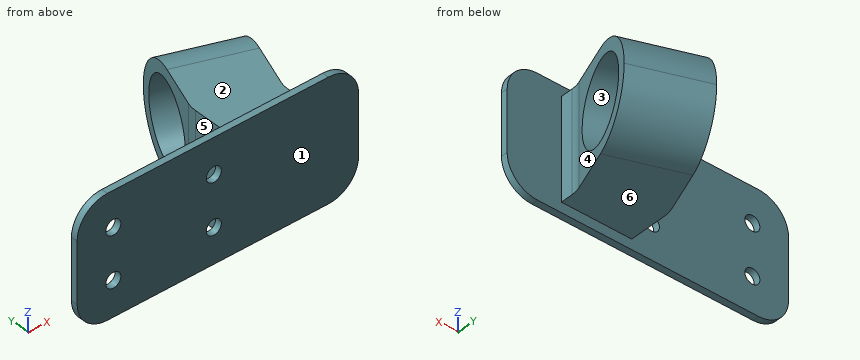
from build123d import *

# Parameters (mm, degrees)
BOSS_EXTRUDE1_DEPTH = 0.65
BOSS_EXTRUDE2_DEPTH = 10
SKETCH9_W           = 7.449244408
SKETCH9_H           = 10
BOSS_EXTRUDE3_DEPTH = 10
CUT_EXTRUDE1_REACH  = 15.344
SKETCH10_R          = 3.85
CUT_EXTRUDE2_REACH  = 2.65
SKETCH6_R           = 0.75
FILLET1_R           = 3


with BuildPart() as part:
    # Sketch1 → Boss-Extrude1 (new body)
    with BuildSketch(Plane(origin=(0, 0, 0), x_dir=(1, 0, 0), z_dir=(0, 1, 0))):
        with BuildLine():
            Line((-11, -6), (11, -6))
            ThreePointArc((11, -6), (13.121320344, -5.121320344), (14, -3))
            Line((14, -3), (14, 3))
            ThreePointArc((14, 3), (13.121320344, 5.121320344), (11, 6))
            Line((11, 6), (-11, 6))
            ThreePointArc((-11, 6), (-13.121320344, 5.121320344), (-14, 3))
            Line((-14, 3), (-14, -3))
            ThreePointArc((-14, -3), (-13.121320344, -5.121320344), (-11, -6))
        make_face()
    extrude(amount=BOSS_EXTRUDE1_DEPTH)

    # Sketch8 → Boss-Extrude2 (add)
    with BuildSketch(Plane.XY.offset(5)):
        Polygon((1.6, 0.65), (1.6, 4.94779164), (8.6, 2.4), (8.6, 0.65), align=None)
    extrude(amount=-BOSS_EXTRUDE2_DEPTH)

    # Sketch9 → Boss-Extrude3 (add)
    with BuildSketch(Plane(origin=(1.777354026, 4.883240053, 0), x_dir=(0.939692621, -0.342020143, 0), z_dir=(0.342020143, 0.939692621, 0))):
        with Locations((3.535885991, 0)):
            Rectangle(SKETCH9_W, SKETCH9_H)
    extrude(amount=BOSS_EXTRUDE3_DEPTH)

    # Sketch10 → Cut-Extrude1 (cut, up to next)
    with BuildSketch(Plane(origin=(-0.177354026, 0.064551586, 0), x_dir=(0, 0, 1), z_dir=(-0.939692621, 0.342020143, 0)), mode=Mode.PRIVATE) as cut_extrude1_sk1:
        with BuildLine():
            Line((5, 15.196635522), (-6.8e-08, 15.196635522))
            ThreePointArc((-6.8e-08, 15.196635522), (3.535533882, 13.732169453), (5, 10.196635522))
            Line((5, 10.196635522), (5, 15.196635522))
        make_face()
    cut_extrude1_tool1 = extrude(cut_extrude1_sk1.sketch, amount=-CUT_EXTRUDE1_REACH, mode=Mode.PRIVATE) & part.part
    add(cut_extrude1_tool1.solids().sort_by_distance((4.63822, 13.295232, 3.88316))[0], mode=Mode.SUBTRACT)
    # Sketch10 → Cut-Extrude1 (cut, up to next)
    with BuildSketch(Plane(origin=(-0.177354026, 0.064551586, 0), x_dir=(0, 0, 1), z_dir=(-0.939692621, 0.342020143, 0)), mode=Mode.PRIVATE) as cut_extrude1_sk2:
        with BuildLine():
            Line((-5, 15.196635522), (-5, 10.196635522))
            ThreePointArc((-5, 10.196635522), (-3.53553393, 13.732169404), (-6.8e-08, 15.196635522))
            Line((-6.8e-08, 15.196635522), (-5, 15.196635522))
        make_face()
    cut_extrude1_tool2 = extrude(cut_extrude1_sk2.sketch, amount=-CUT_EXTRUDE1_REACH, mode=Mode.PRIVATE) & part.part
    add(cut_extrude1_tool2.solids().sort_by_distance((4.63822, 13.295232, -3.88316))[0], mode=Mode.SUBTRACT)
    # Sketch10 → Cut-Extrude1 (cut, up to next)
    with BuildSketch(Plane(origin=(-0.177354026, 0.064551586, 0), x_dir=(0, 0, 1), z_dir=(-0.939692621, 0.342020143, 0)), mode=Mode.PRIVATE) as cut_extrude1_sk3:
        with Locations((0, 10.196635522)):
            Circle(SKETCH10_R)
    cut_extrude1_tool3 = extrude(cut_extrude1_sk3.sketch, amount=-CUT_EXTRUDE1_REACH, mode=Mode.PRIVATE) & part.part
    add(cut_extrude1_tool3.solids().sort_by_distance((3.310101, 9.646255, 0))[0], mode=Mode.SUBTRACT)

    # Sketch6 → Cut-Extrude2 (cut, up to next)
    with BuildSketch(Plane(origin=(0, 0.65, 0), x_dir=(1, 0, 0), z_dir=(0, 1, 0)), mode=Mode.PRIVATE) as cut_extrude2_sk1:
        with Locations((-10.4, 2.5)):
            Circle(SKETCH6_R)
    cut_extrude2_tool1 = extrude(cut_extrude2_sk1.sketch, amount=-CUT_EXTRUDE2_REACH, mode=Mode.PRIVATE) & part.part
    add(cut_extrude2_tool1.solids().sort_by_distance((-10.4, 0.65, -2.5))[0], mode=Mode.SUBTRACT)
    # Sketch6 → Cut-Extrude2 (cut, up to next)
    with BuildSketch(Plane(origin=(0, 0.65, 0), x_dir=(1, 0, 0), z_dir=(0, 1, 0)), mode=Mode.PRIVATE) as cut_extrude2_sk2:
        with Locations((-0.4, 2.5)):
            Circle(SKETCH6_R)
    cut_extrude2_tool2 = extrude(cut_extrude2_sk2.sketch, amount=-CUT_EXTRUDE2_REACH, mode=Mode.PRIVATE) & part.part
    add(cut_extrude2_tool2.solids().sort_by_distance((-0.4, 0.65, -2.5))[0], mode=Mode.SUBTRACT)
    # Sketch6 → Cut-Extrude2 (cut, up to next)
    with BuildSketch(Plane(origin=(0, 0.65, 0), x_dir=(1, 0, 0), z_dir=(0, 1, 0)), mode=Mode.PRIVATE) as cut_extrude2_sk3:
        with Locations((-0.4, -2.5)):
            Circle(SKETCH6_R)
    cut_extrude2_tool3 = extrude(cut_extrude2_sk3.sketch, amount=-CUT_EXTRUDE2_REACH, mode=Mode.PRIVATE) & part.part
    add(cut_extrude2_tool3.solids().sort_by_distance((-0.4, 0.65, 2.5))[0], mode=Mode.SUBTRACT)
    # Sketch6 → Cut-Extrude2 (cut, up to next)
    with BuildSketch(Plane(origin=(0, 0.65, 0), x_dir=(1, 0, 0), z_dir=(0, 1, 0)), mode=Mode.PRIVATE) as cut_extrude2_sk4:
        with Locations((-10.4, -2.5)):
            Circle(SKETCH6_R)
    cut_extrude2_tool4 = extrude(cut_extrude2_sk4.sketch, amount=-CUT_EXTRUDE2_REACH, mode=Mode.PRIVATE) & part.part
    add(cut_extrude2_tool4.solids().sort_by_distance((-10.4, 0.65, 2.5))[0], mode=Mode.SUBTRACT)

    # Fillet1
    fillet1_edges = [part.edges().sort_by_distance(p)[0] for p in [
        (1.6, 4.94779164, 0),
        (8.6, 2.4, 0),
    ]]
    fillet(fillet1_edges, radius=FILLET1_R)


solid = part.part
CAD build for the part. Positions are in the model's coordinates, mm. Face numbers are marked on the shaded views. A direction names the side the tool comes from. Round coordinates to 2 decimals unless told otherwise and drop trailing zeros. Write each loop counter-clockwise with the first axis right and the second up, starting at its lowest first coordinate (ties: lowest second). Pieces come first, ordered by that corner, then holes. Notation, with made-up numbers: M 26,9 L 65,9 A6 ccw 65,14 Z; hole C -32,14.25 d5. An arc over 180 degrees is marked long. Put each result on its own line as item: value. Start each with the question number.
1) Drill centre lines: probe 1 along Z at (x, y) = (-0.4, 0.5); probe 2 along X at (y, z) = (0.45, -2.5); probe 3 along X at (y, z) = (2, 0). Where is each one in solid material? Low to high. Write a range as [from, to].
2) Saw through at D-D, the plane x = -6.5. Write the cut outline in (y, z).
3) Saw through at C-C, the plane z = 2.5. Write the cut outline in (x, y), and give its area (3 significant figures).
4) Saw through at A-A, the plane x = -0.4. Write the cut outline in (y, z).
5) 3-axis set-ups, long thin cutter, end or side, ignore diameter. For the marked faces 4, 5 and 6: which of +Z, -Z, +X, -X, +Y, -Y reach the whole face in a straight line?
6) Saw through at B-B, the plane z = -0.75. Write the cut outline in (x, y), and give its area (3 significant figures).
7) Pin check, flat tips, straight feed: pin 1 Ø0.6 at (y, z) = (1, -1.5) entering from +X; pin 2 Ø4 at (x, y) = (3, 7.5) entering from +Z; pin 3 Ø6 at (x, z) = (-3, 0.5) entering from -Y; pin 4 Ø2 at (x, z) = (-10.4, -2.5) entering from +Y. Stop position of each tip, or through.
8) Pull direction Y, two halves, no side cores. Call the marked faces 1, 2 and 3: pulls with the +Y half, pulls with the -Y half, needs draft (parallel to the pull), parting line crosses it, or undercut.
Resolved:
1. probe 1: [-6, -3.25], [-1.75, 1.75], [3.25, 6]
1. probe 2: [-14, -11.15], [-9.65, -1.15], [0.35, 14]
1. probe 3: [1.6, 8.6]
2. outline: M 0,-6 L 0.65,-6 L 0.65,6 L 0,6 Z
3. outline: M -14,0 L -11.15,0 L -11.15,0.65 L -14,0.65 Z; M -9.65,0 L -1.15,0 L -1.15,0.65 L -9.65,0.65 Z; M 0.35,0 L 14,0 L 14,0.65 L 8.6,0.65 L 8.6,1.87 A3 cw 8.78,2.9 L 9.31,4.35 L 2.31,6.89 L 1.78,5.44 A3 ccw 1.6,4.42 L 1.6,0.65 L 0.35,0.65 Z; M 4.31,12.4 L 11.31,9.85 L 11.79,11.17 L 4.79,13.72 Z
3. area: 63.3 mm²
4. outline: M 0,-6 L 0.65,-6 L 0.65,-3.25 L 0,-3.25 Z; M 0,-1.75 L 0.65,-1.75 L 0.65,1.75 L 0,1.75 Z; M 0,3.25 L 0.65,3.25 L 0.65,6 L 0,6 Z
5. face 4: +Z, -Z, +X
5. face 5: +Z, -Z, -X, +Y
5. face 6: -Z, +X, -X, +Y
6. outline: M -14,0 L 14,0 L 14,0.65 L 8.6,0.65 L 8.6,1.87 A3 cw 8.78,2.9 L 9.02,3.55 L 2.02,6.1 L 1.78,5.44 A3 ccw 1.6,4.42 L 1.6,0.65 L -14,0.65 Z; M 4.6,13.19 L 11.6,10.65 L 12,11.74 L 5,14.29 Z
6. area: 57.2 mm²
7. pin 1: x = 8.6
7. pin 2: z = 5
7. pin 3: y = 0
7. pin 4: y = 0.65
8. face 1: pulls with the -Y half
8. face 2: needs draft
8. face 3: undercut
